Read the model definition and answer for the solid it produces. Units are mm, in the model's axes. A direction names the side the tool comes from. Round coordinates to 2 decimals unless told otherwise and drop trailing zeros. Order: outer loops, then holes, each group sorted by start corner. A loop starts at its lowest first (then second) coordinate and runs counter-clockwise, first axis right, second up. Notation, with made-up numbers: M -13.5,-30.5 L 41.5,-30.5 A19 cw 41.5,6.5 Z; hole C 73.25,19.25 d1. An arc over 180 degrees is marked long. Answer as CSV lines item,"result".
```python
from build123d import *

# Parameters (mm, degrees)
F0_W      = 28
F0_H      = 28
F1_DEPTH  = 10
F3_DEPTH  = 4
F5_DEPTH  = 4
F6_SIZE   = 3
F7_R      = 1.5
F8_R      = 5
F9_R      = 2.5
F10_DEPTH = 2


with BuildPart() as f1:
    # F0 (on Top) → F1 (new body)
    with BuildSketch(Plane.XY):
        with Locations((14, 14)):
            Rectangle(F0_W, F0_H)
    extrude(amount=F1_DEPTH)

    # F2 (on face) → F3 (cut)
    with BuildSketch(Plane.XY.offset(10)):
        with BuildLine():
            ThreePointArc((26, 22), (24.8284271247, 24.8284271247), (22, 26))
            Line((22, 26), (6, 26))
            ThreePointArc((6, 26), (3.1715728753, 24.8284271247), (2, 22))
            Line((2, 22), (2, 6))
            ThreePointArc((2, 6), (3.1715728753, 3.1715728753), (6, 2))
            Line((6, 2), (22, 2))
            ThreePointArc((22, 2), (24.8284271247, 3.1715728753), (26, 6))
            Line((26, 6), (26, 22))
        make_face()
    extrude(amount=-F3_DEPTH, mode=Mode.SUBTRACT)

    # F4 (on face) → F5 (cut)
    with BuildSketch(Plane.XY.offset(6)):
        with BuildLine():
            Line((10, 11), (2, 11))
            Line((2, 11), (2, 6))
            ThreePointArc((2, 6), (3.1715728753, 3.1715728753), (6, 2))
            Line((6, 2), (22, 2))
            ThreePointArc((22, 2), (24.8284271247, 3.1715728753), (26, 6))
            Line((26, 6), (26, 11))
            Line((26, 11), (18, 11))
            Line((18, 11), (18, 17))
            Line((18, 17), (10, 17))
            Line((10, 17), (10, 11))
        make_face()
    extrude(amount=-F5_DEPTH, mode=Mode.SUBTRACT)

    # F6
    f6_edges = [f1.edges().sort_by_distance(p)[0] for p in [
        (0, 0, 5),
        (28, 28, 5),
    ]]
    chamfer(f6_edges, length=F6_SIZE)

    # F7
    f7_edges = [f1.edges().sort_by_distance(p)[0] for p in [
        (2, 11, 4),
        (10, 17, 4),
        (18, 17, 4),
        (26, 11, 4),
    ]]
    fillet(f7_edges, radius=F7_R)

    # F8
    f8_edges = [f1.edges().sort_by_distance(p)[0] for p in [
        (0, 28, 5),
    ]]
    fillet(f8_edges, radius=F8_R)

    # F9 (on face) → F10 (cut)
    with BuildSketch(Plane.XY.offset(6)):
        with BuildLine():
            Line((11.5, 20), (11.5, 17))
            Line((11.5, 17), (16.5, 17))
            Line((16.5, 17), (16.5, 20))
            Line((16.5, 20), (21, 20))
            ThreePointArc((21, 20), (22.0606601718, 20.4393398282), (22.5, 21.5))
            Line((22.5, 21.5), (22.5, 23))
            ThreePointArc((22.5, 23), (22.0606601718, 24.0606601718), (21, 24.5))
            Line((21, 24.5), (7, 24.5))
            ThreePointArc((7, 24.5), (5.9393398282, 24.0606601718), (5.5, 23))
            Line((5.5, 23), (5.5, 21.5))
            ThreePointArc((5.5, 21.5), (5.9393398282, 20.4393398282), (7, 20))
            Line((7, 20), (11.5, 20))
        make_face()
        with Locations((22, 15.75)):
            Circle(F9_R)
        with Locations((6, 15.75)):
            Circle(F9_R)
    extrude(amount=-F10_DEPTH, mode=Mode.SUBTRACT)


solid = f1.part
```
Item 1: Determine the mould class of faces 3 (the face through (28, 12, 5)), 4 (the face through (2, 27, 5)), 5 (the face through (26, 12, 7)) for opening direction Y: +Y half, -Y half, draft (parallel to the pull), parting line (faces both ways), or undercut.
Ans:
face 3,"draft"
face 4,"+Y half"
face 5,"undercut"
Item 2: A cutting plane is placed at C-C, the plane z = 4.75. Give the number of separate pieces and of enclosed holes in the cut face, and give its area (3 significant figures).
Ans:
separate pieces,"1"
enclosed holes,"3"
area,"386 mm2"
Item 3: A cutting plane is placed at D-D, the plane y = 6.75. Determine the outline of the cut face in (x, z), and give its area (3 significant figures).
Ans:
outline,"M 0,0 L 28,0 L 28,10 L 26,10 L 26,2 L 2,2 L 2,10 L 0,10 Z"
area,"88.0 mm2"
Item 4: Flat-ended cylindrical pins translate along their axes: pin 1 (1.5 mm diameter, centred on x = 17, y = 21.5, fed in from +Z); pin 2 (1 mm diameter, centred on x = 21.5, y = 12.5, fed in from -Z); pin 3 (4 mm diameter, centred on x = 21, y = 16, fed in from +Z). Find the tip coordinate at first contact, or state that the pin passes through.
Ans:
pin 1,"z = 4"
pin 2,"z = 0"
pin 3,"z = 6"
Item 5: A cutting plane is placed at B-B, the plane x = 20.5. Determine the outline of the cut face in (y, z), and give its area (3 significant figures).
Ans:
outline,"M 0,0 L 28,0 L 28,10 L 26,10 L 26,6 L 24.5,6 L 24.5,4 L 20,4 L 20,6 L 17.75,6 L 17.75,4 L 13.75,4 L 13.75,6 L 11,6 L 11,2 L 2,2 L 2,10 L 0,10 Z"
area,"131 mm2"
Item 6: Find the intervals of material crossed by probe 1 along X at (y, z) = (6, 4.25); probe 2 along Y at (x, z) = (6, 5.5); probe 3 along X at (y, z) = (21.5, 5), in increasing order. Write a range as [from, to].
Ans:
probe 1,"[0, 2], [26, 28]"
probe 2,"[0, 2], [11, 13.25], [18.25, 20.38], [24.12, 28]"
probe 3,"[0, 5.5], [22.5, 28]"
Item 7: A cutting plane is placed at A-A, the plane z = 7. Determine the outline of the cut face in (x, y).
Ans:
outline,"M 0,3 L 3,0 L 28,0 L 28,25 L 25,28 L 5,28 A5 ccw 0,23 Z; hole M 2,6 A4 ccw 6,2 L 22,2 A4 ccw 26,6 L 26,22 A4 ccw 22,26 L 6,26 A4 ccw 2,22 Z"
Item 8: A tool of negligible diameter and unlimited length cuts with its end or side. For faces 1 (the face through (6, 16, 4)), 2 (the face through (15, 28, 5)), from which of +Z, -Z, +X, -X, +Y, -Y can it reach the whole face along a straight path? Write none if from no direction.
Ans:
face 1,"+Z"
face 2,"+Z, -Z, +X, -X, +Y"
